Geometry: final body of the model. Coordinates: model frame, mm. A direction names the side the tool comes from. Give positions to 0.01 mm unless a question says otherwise; leave off trailing zeros. Loops run counter-clockwise (first coordinate to the right, second up) from the corner with the lowest first, then second, coordinate; pieces in that order, holes last. Notation, with made-up numbers: M 0.25,-7.5 L 54.25,-7.5 A10 cw 54.25,9.5 Z; hole C 3,20 d3. An arc over 180 degrees is marked long. Put each result on its own line as item: value.
```python
from build123d import *

# Parameters (mm, degrees)
PAD_DEPTH    = 5
SKETCH001_W  = 2.5
SKETCH001_H  = 4.4
POCKET_DEPTH = 8
SKETCH002_R  = 1.25
HOLE_DEPTH   = 7
HOLE_TIPS_R  = 1.25


with BuildPart() as part:
    # Sketch → Pad (new body, symmetric)
    with BuildSketch(Plane.XY):
        with BuildLine():
            Line((45, 12), (45, 20))
            Line((45, 20), (-45, 20))
            Line((-45, 20), (-44, 12))
            Line((-44, 12), (-37.5, 12))
            Line((-37.5, 12), (-37.5, 10.7))
            Line((-37.5, 10.7), (-41.3, 10.7))
            Line((-41.3, 10.7), (-41.3, 7.7))
            Line((-41.3, 7.7), (-45.8, 7.7))
            Line((-45.8, 7.7), (-45.8, 1.8))
            Line((-41.3, 1.8), (-45.8, 1.8))
            Line((-18.65, 1.8), (-41.3, 1.8))
            Line((-18.086075, 2.472059), (-18.65, 1.8))
            ThreePointArc((-18.086075, 2.472059), (-17.104232, 4.013245), (-16.554732, 5.756036))
            Line((-16.45, 6.35), (-16.554732, 5.756036))
            Line((-16.45, 6.35), (-17.35, 6.35))
            ThreePointArc((-17.65, 6.65), (-17.562132, 6.437868), (-17.35, 6.35))
            Line((-17.65, 6.65), (-17.65, 7.5))
            Line((-17.65, 7.5), (-16.45, 7.5))
            Line((-16.45, 7.5), (-17.5, 8.9))
            Line((-17.5, 8.9), (-17.5, 9.4))
            Line((-17.5, 9.4), (-13.7, 9.4))
            Line((-13.7, 9.4), (-13.7, 12))
            Line((-13.7, 12), (-7, 12))
            Line((-7, 12), (-7, 7.5))
            Line((-7, 7.5), (-1.2, 7.5))
            ThreePointArc((3.912237, 5.991471), (1.465081, 7.114997), (-1.2, 7.5))
            Line((3.912237, 5.991471), (7.271446, 3.819901))
            ThreePointArc((7.5, 3.4), (7.43916, 3.639036), (7.271446, 3.819901))
            Line((7.5, 3.4), (7.5, 3.2))
            ThreePointArc((7.5, 3.2), (7.646447, 2.846447), (8, 2.7))
            Line((8, 2.7), (9.2, 2.7))
            Line((9.2, 2.7), (9.2, 1))
            Line((9.2, 1), (11.7, 1))
            ThreePointArc((11.7, 1), (12.265685, 1.234315), (12.5, 1.8))
            Line((12.5, 1.8), (12.5, 3))
            Line((12.5, 3), (11.5, 3))
            Line((11.5, 3), (11.5, 4))
            Line((11.5, 4), (12.5, 4))
            Line((12.5, 4), (12.2, 5.220135))
            Line((12.2, 5.220135), (9.9, 12))
            Line((9.9, 12), (10.9, 12))
            Line((10.9, 12), (12.426579, 7.5))
            Line((12.426579, 7.5), (17.65, 7.5))
            Line((17.65, 7.5), (17.65, 6.65))
            ThreePointArc((17.35, 6.35), (17.562132, 6.437868), (17.65, 6.65))
            Line((17.35, 6.35), (16.45, 6.35))
            Line((16.45, 6.35), (16.45, 5.55))
            ThreePointArc((16.45, 5.55), (16.655025, 5.055025), (17.15, 4.85))
            Line((17.15, 4.85), (19.45, 4.85))
            ThreePointArc((19.45, 4.85), (20.864214, 5.435786), (21.45, 6.85))
            Line((21.45, 6.85), (21.45, 12))
            Line((45, 12), (21.45, 12))
        make_face()
        with BuildLine():
            Line((-5.7, 12), (-5.7, 8.8))
            Line((-5.7, 8.8), (-1.2, 8.8))
            ThreePointArc((4.617998, 7.083214), (1.833004, 8.361846), (-1.2, 8.8))
            Line((4.617998, 7.083214), (7.5, 5.220135))
            Line((7.5, 5.220135), (10, 5.220135))
            Line((10, 5.220135), (9.3, 12))
            Line((9.3, 12), (-5.7, 12))
        make_face(mode=Mode.SUBTRACT)
        Polygon((-36.2, 12), (-36.2, 9.4), (-40, 9.4), (-40, 3.1), (-18.8, 3.1), (-18.8, 10.7), (-15, 10.7), (-15, 12), align=None, mode=Mode.SUBTRACT)
    extrude(amount=PAD_DEPTH, both=True)

    # Sketch001 (on Face67 of Pad) → Pocket (cut)
    with BuildSketch(Plane.XY.offset(5)):
        with Locations((-43.05, 5.5)):
            Rectangle(SKETCH001_W, SKETCH001_H)
    extrude(amount=-POCKET_DEPTH, mode=Mode.SUBTRACT)

    # Sketch002 (on Face13 of Pocket) → Hole (cut)
    with BuildSketch(Plane(origin=(0, 20, 0), x_dir=(-1, 0, 0), z_dir=(0, 1, 0))):
        Circle(SKETCH002_R)
        with Locations((-37.5, 0)):
            Circle(SKETCH002_R)
        with Locations((37.5, 0)):
            Circle(SKETCH002_R)
    extrude(amount=-HOLE_DEPTH, mode=Mode.SUBTRACT)

    # Hole tips → Hole tip 1 section 0
    with BuildSketch(Plane(origin=(0, 13, 0), x_dir=(-1, 0, 0), z_dir=(0, 1, 0)), mode=Mode.PRIVATE) as hole_tip_1_s0:
        Circle(HOLE_TIPS_R)
    loft([hole_tip_1_s0.sketch, Vertex(0, 12.248924, 0)], mode=Mode.SUBTRACT)

    # Hole tips → Hole tip 2 section 0
    with BuildSketch(Plane(origin=(0, 13, 0), x_dir=(-1, 0, 0), z_dir=(0, 1, 0)), mode=Mode.PRIVATE) as hole_tip_2_s0:
        with Locations((-37.5, 0)):
            Circle(HOLE_TIPS_R)
    loft([hole_tip_2_s0.sketch, Vertex(37.5, 12.248924, 0)], mode=Mode.SUBTRACT)

    # Hole tips → Hole tip 3 section 0
    with BuildSketch(Plane(origin=(0, 13, 0), x_dir=(-1, 0, 0), z_dir=(0, 1, 0)), mode=Mode.PRIVATE) as hole_tip_3_s0:
        with Locations((37.5, 0)):
            Circle(HOLE_TIPS_R)
    loft([hole_tip_3_s0.sketch, Vertex(-37.5, 12.248924, 0)], mode=Mode.SUBTRACT)


solid = part.part
```
Item 1: Line query: probe 1 along Z at (x, y) = (37.5, 16); probe 2 along X at (y, z) = (18.5, 0.5); probe 3 along Y at (x, z) = (9, -1.25). Output: solid intervals per line, ascending. Write a range as [from, to].
Output values:
probe 1: [-5, -1.25], [1.25, 5]
probe 2: [-44.81, -38.65], [-36.35, -1.15], [1.15, 36.35], [38.65, 45]
probe 3: [2.7, 5.22], [12, 20]
Item 2: Section A-A on x = -23. Output: boundary loops of the cut face in (y, z).
Output values:
outline: M 1.8,-5 L 3.1,-5 L 3.1,5 L 1.8,5 Z; M 12,-5 L 20,-5 L 20,5 L 12,5 Z
Item 3: Section B-B on y = 15.75. Output: boundary loops of the cut face in (x, z), then the cut area to 3 significant figures.
Output values:
outline: M -44.47,-5 L 45,-5 L 45,5 L -44.47,5 Z; hole C -37.5,0 d2.5; hole C 0,0 d2.5; hole C 37.5,0 d2.5
area: 880 mm²
Item 4: Section C-C on z = -2.25. Count the separate pieces of the cut face and the enclosed holes in it, then the cut area to 3 significant figures.
Output values:
separate pieces: 1
enclosed holes: 2
area: 903 mm²
Item 5: Set-up query: faces 1 (the flat face through (18, 4.85, 0)), 2 (the flat face through (-41.3, 9, 0)), 3 (the cylindrical face through (0.27, 16.55, -1.22)), 4 (the flat face through (9.655, 8.563, 0.07)), 5 (the flat face through (-7, 10, 0)). Return all of +Z, -Z, +X, -X, +Y, -Y with unobstructed straight access to the full face (end or side cutting, diameter ignored); none if empty.
Output values:
face 1: +Z, -Z, +X, -Y
face 2: +Z, -Z, -X
face 3: +Y
face 4: +Z, -Z
face 5: +Z, -Z, -Y
Item 6: Pin query (flat end, axial travel): pin 1 Ø3 at (x, z) = (-37.5, 0) entering from -Y; pin 2 Ø1.4 at (y, z) = (11.5, -0.5) entering from -X (3 decimals); pin 3 Ø0.8 at (y, z) = (11.5, 1) entering from +X. Return the tip coordinate at first contact, or that it passes through.
Output values:
pin 1: y = 1.8
pin 2: x = -44.025
pin 3: x = 21.45
Item 7: Mould query, pull axis Y, two halves, no side actions, for faces 6 (the cylindrical face through (1.501, 7.104, 0.07)), 7 (the flat face through (-41, 12, 0)), 8 (the flat face through (-1, 13, -5)), 9 (the flat face through (-44.3, 5, 1)). Classes: pulls with the +Y half, pulls with the -Y half, needs draft (parallel to the pull), parting line crosses it, or undercut.
Output values:
face 6: pulls with the -Y half
face 7: undercut
face 8: needs draft
face 9: undercut
Item 8: Section D-D on x = 5.5. Output: boundary loops of the cut face in (y, z).
Output values:
outline: M 4.97,-5 L 6.51,-5 L 6.51,5 L 4.97,5 Z; M 12,-5 L 20,-5 L 20,5 L 12,5 Z
